CAD build for the part. Positions are in the model's coordinates, mm. Face numbers are marked on the shaded views. A direction names the side the tool comes from. Coordinates: 2 decimals unless noted, no trailing zeros. Write each loop counter-clockwise with the first axis right and the second up, starting at its lowest first coordinate (ties: lowest second). Pieces come first, ordered by that corner, then holes.
```python
from build123d import *

# Parameters (mm, degrees)
F1_DEPTH = 12.7
F3_DEPTH = 25.4
F4_SIZE  = 0.508
F6_W     = 14.2258834094
F6_H     = 10.6622967869
F7_DEPTH = 50.8


with BuildPart() as f1:
    # F0 (on Top) → F1 (new body)
    with BuildSketch(Plane.XY):
        with BuildLine():
            Line((15.24, -31.75), (15.24, 31.75))
            Line((15.24, 31.75), (-15.24, 31.75))
            Line((-15.24, 31.75), (-15.24, -31.75))
            ThreePointArc((-15.24, -31.75), (-10.7763073453, -20.9736926547), (0, -16.51))
            ThreePointArc((0, -16.51), (10.7763073453, -20.9736926547), (15.24, -31.75))
        make_face()
        with BuildLine():
            ThreePointArc((-15.24, -31.75), (0, -46.99), (15.24, -31.75))
            Line((15.24, -31.75), (0, -31.75))
            Line((0, -31.75), (-15.24, -31.75))
        make_face()
        with BuildLine():
            Line((0, -31.75), (15.24, -31.75))
            ThreePointArc((15.24, -31.75), (10.7763073453, -20.9736926547), (0, -16.51))
            Line((0, -16.51), (0, -31.75))
        make_face()
        with BuildLine():
            ThreePointArc((0, -16.51), (-10.7763073453, -20.9736926547), (-15.24, -31.75))
            Line((-15.24, -31.75), (0, -31.75))
            Line((0, -31.75), (0, -16.51))
        make_face()
    extrude(amount=F1_DEPTH)

    # F2 (on Top) → F3 (cut)
    with BuildSketch(Plane.XY):
        with BuildLine():
            ThreePointArc((10.16, -31.75), (7.1842048969, -24.5657951031), (0, -21.59))
            Line((0, -21.59), (0, -31.75))
            Line((0, -31.75), (10.16, -31.75))
        make_face()
        with BuildLine():
            Line((0, -31.75), (0, -21.59))
            ThreePointArc((0, -21.59), (-7.1842048969, -38.9342048969), (10.16, -31.75))
            Line((10.16, -31.75), (0, -31.75))
        make_face()
    extrude(amount=F3_DEPTH, mode=Mode.SUBTRACT)

    # F4
    f4_edges = [f1.edges().sort_by_distance(p)[0] for p in [
        (-15.24, 0, 12.7),
        (-15.24, 0, 0),
        (0, -41.91, 12.7),
        (0, -41.91, 0),
    ]]
    chamfer(f4_edges, length=F4_SIZE)

    # F6 (on offset) → F7 (cut)
    with BuildSketch(Plane.XZ.offset(-31.75)):
        with Locations((7.1129417047, 6.336113438)):
            Rectangle(F6_W, F6_H)
        with Locations((-7.1129417047, 6.336113438)):
            Rectangle(F6_W, F6_H)
    extrude(amount=F7_DEPTH, mode=Mode.SUBTRACT)


solid = f1.part
```
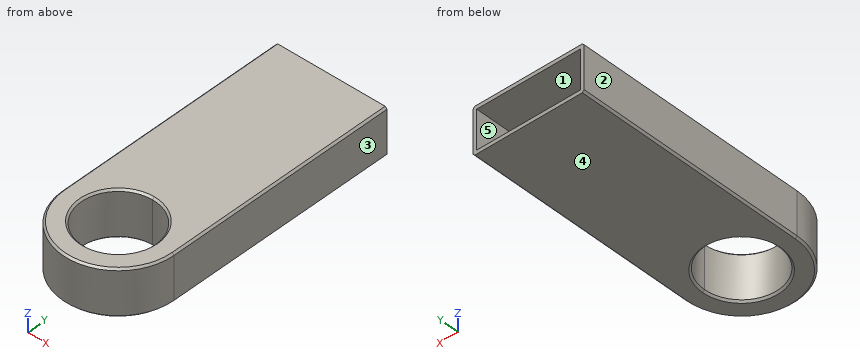
Item 1: Flat gauge pins, fed straight in: pin 1 Ø1.5 at (x, z) = (1.5, 5.5) entering from -Y; pin 2 Ø5.5 at (x, z) = (2, 7.5) entering from +Y. Where does each tip first touch, or does it go through?
Item 2: Saw through at B-B, the plane y = 7. Write the cut outline in (x, z), and give its area (3 significant figures).
Item 3: Two-plate mould, pull along Z, no slides. Class the marked faces 3, 4 and 5: +Z half, -Z half, draft (parallel to the pull), parting line (faces both ways), or undercut.
Item 4: Which spindle directions (+Z, -Z, +X, -X, +Y, -Y) get a long thin tool onto all of the face, cutting with end or side? Do the marked faces 1 and 2. Say none if no direction does.
Item 5: Wall check: line 1 along Y through (x, z) = (0, 5); line 2 along X through (y, z) = (-13.5, 4.5); line 3 along Z through (x, y) = (-10, -7.5). Give the ranges that are in metal, low to high.
Item 6: Saw through at A-A, the plane z = 9.5. Write the cut outline in (x, y).
Working result:
1. pin 1: stops at y = -46.97
1. pin 2: stops at y = -19.05
2. outline: (-15.24, 0.51) - (-14.73, 0) - (14.73, 0) - (15.24, 0.51) - (15.24, 12.19) - (14.73, 12.7) - (-14.73, 12.7) - (-15.24, 12.19) - close; hole (-14.23, 1) - (14.23, 1) - (14.23, 11.67) - (-14.23, 11.67) - close
2. area: 83.2 mm2
3. face 3: draft
3. face 4: -Z half
3. face 5: undercut
4. face 1: +Y
4. face 2: +Z, -Z, -X, +Y, -Y
5. line 1: y = -46.99 to -41.91, -21.59 to -19.05
5. line 2: x = -15.24 to -14.23, 14.23 to 15.24
5. line 3: z = 0 to 1, 11.67 to 12.7
6. outline: (-15.24, -31.75) arc R15.24 ccw to (15.24, -31.75) - (15.24, 31.75) - (14.23, 31.75) - (14.23, -19.05) - (-14.23, -19.05) - (-14.23, 31.75) - (-15.24, 31.75) - close; hole circle Ø20.32 at (0, -31.75)
